Geometry: see drawing. Coordinates: mm, zero at the bounding-box minimum. Coordinates: 2 decimals unless noted, no trailing zeros.
Item 1: Section B-B on y = 4. State how many separate pieces and enclosed holes the cut face has, then the cut area to 3 significant figures.
Item 2: Mould query, pull axis Y, two halves, no side actions, for the marked faces 1, 2, 3 and 4. Classes: released by +Y, released by -Y, zero draft, split by the parting line, or undercut.
Item 3: Contact query for a flat-ended pin moving along its axis: P1, Ø4, axis at y = 4, z = 20.34, coming from the +X side. Output: stop coordinate, or through.
Item 4: Ray query, line 1 (Z direction, x = 7, y = 1) (1 decimal); line 2 (Z direction, x = 12, y = 6.75) (1 decimal); line 3 (Z direction, x = 13, y = 4.25) (1 decimal). Return the intervals inside material, ascending.
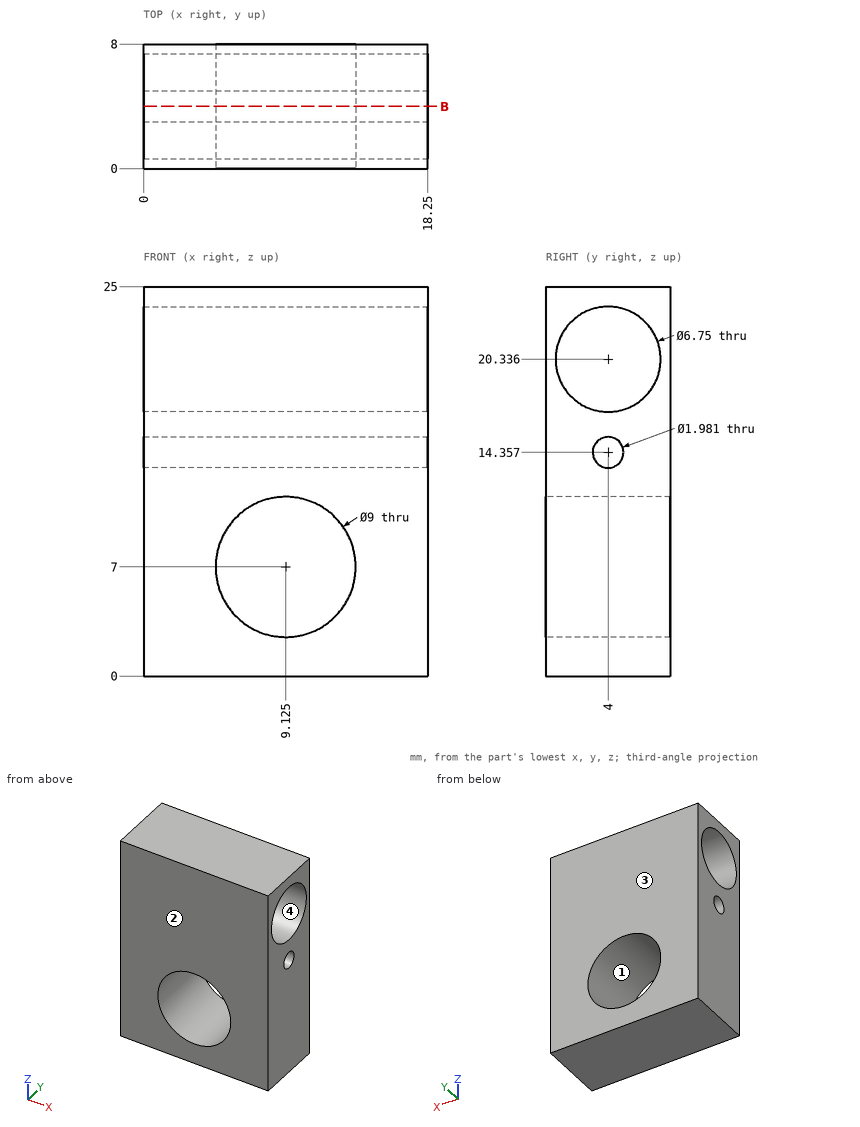
Answer list:
1. separate pieces: 3
1. enclosed holes: 1
1. area: 233 mm2
2. face 1: zero draft
2. face 2: released by -Y
2. face 3: released by +Y
2. face 4: undercut
3. P1: passes through
4. line 1: z = 0 to 3, 11 to 18.8, 21.9 to 25
4. line 2: z = 0 to 3.5, 10.5 to 18.4, 22.3 to 25
4. line 3: z = 0 to 4.7, 9.3 to 13.4, 15.3 to 17, 23.7 to 25
